Check sheet for the modelled part. Datum: model origin and axes. Units: mm. Round coordinates to 2 decimals unless told otherwise and drop trailing zeros. One line per item, written item: value. Start each with the question number.
1. Material ranges on L1, parallel to Y at x = 18.5, z = 0.1; L2, parallel to X at y = 22, z = 0.4; L3, parallel to Y at x = 20, z = 0.5, recorded low to high.
2. Go/stop test with a flat-tipped pin: pin 1 (5.5 mm diameter, centred on x = -18.26, y = 24.61, fed in from +Z). Record where the tip stops, or that it passes through.
3. Cross-section at A-A on x = -16.5. Count the separate pieces of the cut face and the enclosed holes in it, then the cut area to 3 significant figures.
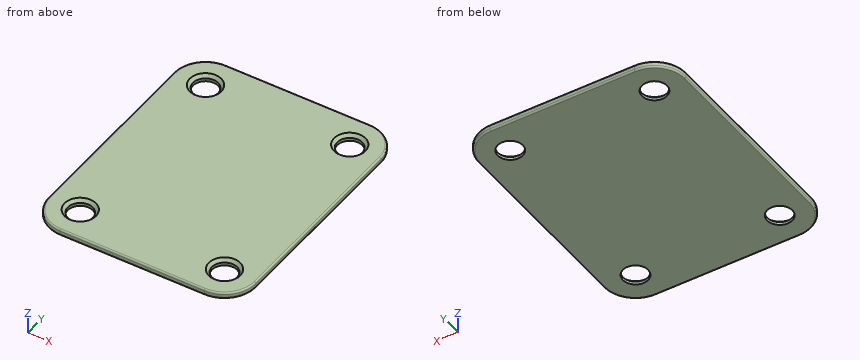
from build123d import *

# Parameters (mm, degrees)
F0_R     = 3.175
F1_DEPTH = 1.5875
F2_R     = 0.396875
F3_SIZE  = 0.79375


with BuildPart() as f1:
    # F0 (on Top) → F1 (new body)
    with BuildSketch(Plane.XY):
        with BuildLine():
            Line((18.25625, 32.54375), (-18.25625, 32.54375))
            ThreePointArc((-18.25625, 32.54375), (-23.86891, 30.21891), (-26.19375, 24.60625))
            Line((-26.19375, 24.60625), (-26.19375, -24.60625))
            ThreePointArc((-26.19375, -24.60625), (-23.86891, -30.21891), (-18.25625, -32.54375))
            Line((-18.25625, -32.54375), (18.25625, -32.54375))
            ThreePointArc((18.25625, -32.54375), (23.86891, -30.21891), (26.19375, -24.60625))
            Line((26.19375, -24.60625), (26.19375, 24.60625))
            ThreePointArc((26.19375, 24.60625), (23.86891, 30.21891), (18.25625, 32.54375))
        make_face()
        with Locations((-18.25625, -24.60625)):
            Circle(F0_R, mode=Mode.SUBTRACT)
        with Locations((18.25625, -24.60625)):
            Circle(F0_R, mode=Mode.SUBTRACT)
        with Locations((-18.25625, 24.60625)):
            Circle(F0_R, mode=Mode.SUBTRACT)
        with Locations((18.25625, 24.60625)):
            Circle(F0_R, mode=Mode.SUBTRACT)
    extrude(amount=F1_DEPTH)

    # F2
    f2_edges = [f1.edges().sort_by_distance(p)[0] for p in [
        (-18.25625, -32.54375, 0.79375),
        (18.25625, -32.54375, 0.79375),
        (0, -32.54375, 0),
        (0, -32.54375, 1.5875),
        (26.19375, -24.60625, 0.79375),
        (23.86891, -30.21891, 0),
        (23.86891, -30.21891, 1.5875),
        (26.19375, 24.60625, 0.79375),
        (26.19375, 0, 0),
        (26.19375, 0, 1.5875),
        (-26.19375, -24.60625, 0.79375),
        (-23.86891, -30.21891, 0),
        (-23.86891, -30.21891, 1.5875),
        (-26.19375, 24.60625, 0.79375),
        (-26.19375, 0, 0),
        (-26.19375, 0, 1.5875),
        (-18.25625, 32.54375, 0.79375),
        (-23.86891, 30.21891, 0),
        (-23.86891, 30.21891, 1.5875),
        (18.25625, 32.54375, 0.79375),
        (0, 32.54375, 0),
        (0, 32.54375, 1.5875),
        (23.86891, 30.21891, 0),
        (23.86891, 30.21891, 1.5875),
    ]]
    fillet(f2_edges, radius=F2_R)

    # F3
    f3_edges = [f1.edges().sort_by_distance(p)[0] for p in [
        (15.08125, -24.60625, 1.5875),
        (-21.43125, -24.60625, 1.5875),
        (-21.43125, 24.60625, 1.5875),
        (15.08125, 24.60625, 1.5875),
    ]]
    chamfer(f3_edges, length=F3_SIZE)


solid = f1.part
Taken from the geometry:
1. L1: y = -32.41 to -27.77, -21.44 to 21.44, 27.77 to 32.41
1. L2: x = -26.19 to -20.07, -16.44 to 16.44, 20.07 to 26.19
1. L3: y = -32.35 to -27.26, -21.95 to 21.95, 27.26 to 32.35
2. pin 1: passes through
3. separate pieces: 3
3. enclosed holes: 0
3. area: 84.9 mm2
